Part model, mm, in its own coordinate system. Face numbers are marked on the shaded views. A direction names the side the tool comes from. Give positions to 0.01 mm unless a question says otherwise; leave off trailing zeros. Order: outer loops, then holes, each group sorted by start corner. A loop starts at its lowest first (then second) coordinate and runs counter-clockwise, first axis right, second up.
1. Which spindle directions (+Z, -Z, +X, -X, +Y, -Y) get a long thin tool onto all of the face, cutting with end or side? Do the marked faces 1 and 2. Say none if no direction does.
2. Slice it at D-D on x = 15. List the corners of the cut face in (y, z), and give its area (3 significant figures).
3. Slice it at B-B on y = 35. List the corners of the cut face in (x, z).
4. Probe line 1 (Y direction, x = 35, z = 18); line 2 (Y direction, x = -33, z = 22). List the from-to ranges inside material, lowest first.
5. Mould opens along Y. For the marked faces 3, 4 and 5 say: +Y half, -Y half, draft (parallel to the pull), parting line (faces both ways), or undercut.
6. Slice it at C-C on z = 17.5. List the corners of the cut face in (x, y), and give its area (3 significant figures).
7. Drop flat-ended pins along their axis: pin 1 Ø11 at (x, y) = (-33, 35.5) entering from +Z; pin 2 Ø3 at (x, y) = (36.5, -35) entering from +Z; pin 3 Ø9 at (x, y) = (-35, 35) entering from -Z. Give the stop position or say it passes through.
8. Slice it at A-A on x = 0. List the corners of the cut face in (y, z).
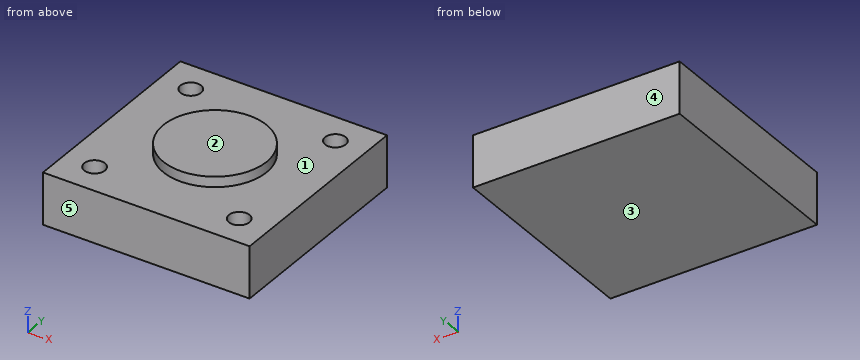
from build123d import *

# Parameters (mm, degrees)
F0_W     = 100
F0_H     = 100
F1_DEPTH = 25
F2_R     = 25
F3_DEPTH = 5
F4_R     = 5
F5_DEPTH = 15


with BuildPart() as f1:
    # F0 (on Top) → F1 (new body)
    with BuildSketch(Plane.XY):
        Rectangle(F0_W, F0_H)
    extrude(amount=F1_DEPTH)

    # F2 (on face) → F3 (join)
    with BuildSketch(Plane.XY.offset(25)):
        Circle(F2_R)
    extrude(amount=F3_DEPTH)

    # F4 (on face) → F5 (cut)
    with BuildSketch(Plane.XY.offset(25)):
        with Locations((-35, -35)):
            Circle(F4_R)
        with Locations((-35, 35)):
            Circle(F4_R)
        with Locations((35, 35)):
            Circle(F4_R)
        with Locations((35, -35)):
            Circle(F4_R)
    extrude(amount=-F5_DEPTH, mode=Mode.SUBTRACT)


solid = f1.part
Data:
1. face 1: +Z
1. face 2: +Z, +X, -X, +Y, -Y
2. outline: (-50, 0) - (50, 0) - (50, 25) - (20, 25) - (20, 30) - (-20, 30) - (-20, 25) - (-50, 25) - close
2. area: 2,700 mm2
3. outline: (-50, 0) - (50, 0) - (50, 25) - (40, 25) - (40, 10) - (30, 10) - (30, 25) - (-30, 25) - (-30, 10) - (-40, 10) - (-40, 25) - (-50, 25) - close
4. line 1: y = -50 to -40, -30 to 30, 40 to 50
4. line 2: y = -50 to -39.58, -30.42 to 30.42, 39.58 to 50
5. face 3: draft
5. face 4: +Y half
5. face 5: -Y half
6. outline: (-50, -50) - (50, -50) - (50, 50) - (-50, 50) - close; hole circle Ø10 at (-35, -35); hole circle Ø10 at (-35, 35); hole circle Ø10 at (35, -35); hole circle Ø10 at (35, 35)
6. area: 9,690 mm2
7. pin 1: stops at z = 25
7. pin 2: stops at z = 10
7. pin 3: stops at z = 0
8. outline: (-50, 0) - (50, 0) - (50, 25) - (25, 25) - (25, 30) - (-25, 30) - (-25, 25) - (-50, 25) - close
